The model under review builds one solid part; all positions refer to its coordinate system, in mm. Face numbers are marked on the shaded views. A direction names the side the tool comes from. Round coordinates to 2 decimals unless told otherwise and drop trailing zeros. Order: outer loops, then holes, each group sorted by start corner. A loop starts at its lowest first (then second) coordinate and runs counter-clockwise, first axis right, second up. Notation, with made-up numbers: M -33,-22.5 L 22,-22.5 A24 ccw 22,10.5 Z; hole C 87,19 d5. An arc over 180 degrees is marked long. Answer as a JSON object with one key per item and string values. Group by question number.
1. Add section C-C on y = -5.5. State the section outline as (x, z) points.
2. Add section A-A on x = 8. State the section outline as (y, z) points.
3. Add section D-D on z = -26. State the section outline as (x, y) points, and give its area (3 significant figures).
4. Clearance check with flat-ended pins moving along their axes: P1, Ø3, axis at x = 33, z = -48.5, coming from the -Y side; P2, Ø6.5, axis at x = 76.5, z = -55.5, coming from the -Y side; P3, Ø2, axis at x = 25, y = 2, coming from the +Z side. State where each tip first meets the part, or that it passes through.
5. Add section B-B on y = 3.5. State the section outline as (x, z) points.
6. Machinability: for the marked faces 1 and 2, which of the approach directions +Z, -Z, +X, -X, +Y, -Y give a long, thin tool a straight path to every point of the face, cutting with its end or side? Answer none if there is none.
7. To check wall thickness, follow probe 1 along Z at (x, y) = (42, 4); probe 2 along Y at (x, z) = (53, -52); probe 3 along X at (y, z) = (0.5, -25.5). State the ranges of each line that lie inside material, in increasing order. Write a range as [from, to].
Autodesk Inventor part; units mm, degrees
ref_plane "YZ Plane" through (0, 0, 0) normal (1, 0, 0) x (0, 1, 0)
ref_plane "XZ Plane" through (0, 0, 0) normal (0, 1, 0) x (-1, 0, 0)
ref_plane "XY Plane" through (0, 0, 0) normal (0, 0, 1) x (1, 0, 0)
sketch "Boceto1" plane through (0, 0, 0) normal (0, 1, 0) x (-1, 0, 0)
  line L0 (0, -100) -> (0, 0)
  line L1 (-76, -48) -> (-24, -48)
  line L2 (-24, -64) -> (-76, -64)
  arc A0 (-16, -100) -> (0, -100) centre (-8, -100) ccw
  arc A1 (0, 0) -> (-16, 0) centre (-8, 0) ccw
  arc A2 (-76, -48) -> (-76, -64) centre (-76, -56) ccw
  line L3 (-16, 0) -> (-16, -40)
  line L4 (-16, -72) -> (-16, -100)
  arc A3 (-24, -48) -> (-16, -40) centre (-24, -40) ccw
  arc A4 (-16, -72) -> (-24, -64) centre (-24, -72) ccw
  circle A5 centre (-8, 0) radius 4
  circle A6 centre (-8, -100) radius 4
  circle A7 centre (-76, -56) radius 4
  circle A8 centre (-76, -58) radius 0.5
  circle A9 centre (-76, -54) radius 0.5
  circle A10 centre (-8, -100) radius 2
  circle A11 centre (-8, 0) radius 2
  point P0 (-16, -48)
  dimension "d0" = 16
  dimension "d1" = 100
  dimension "d2" = 60
  dimension "d3" = 16
  dimension "d6" = 8
  dimension "d7" = 8
  dimension "d8" = 8
  dimension "d9" = 8
  dimension "d10" = 8
  dimension "d11" = 8
  dimension "d12" = 8
  dimension "d13" = 1
  dimension "d14" = 1
  dimension "d15" = 2
  dimension "d16" = 2
  dimension "d17" = 4
  dimension "d18" = 4
extrude "Extrusión1" add sketch "Boceto1" along normal blind 5 contours A0 L4 A4 L2 A2 L1 A3 L3 A1 L0 | A5 | A6 | A7 | A8 | A9 | A10 | A11
sketch "Boceto4" plane through (0, 0, 0) normal (0, -1, 0) x (1, 0, 0)
  point P0 (0, 0)
extrude "Extrusión3" add sketch "Boceto1" against normal blind 14 contours A10 | A11
sketch "Boceto5" plane through (0, 0, 0) normal (0, -1, 0) x (1, 0, 0)
  point P0 (0, 0)
extrude "Extrusión4" add sketch "Boceto1" against normal blind 12 contours A8 | A9
sketch "Boceto6" plane through (0, 0, 0) normal (0, -1, 0) x (1, 0, 0)
  point P0 (0, 0)
extrude "Extrusión5" add sketch "Boceto1" against normal blind 10 contours A5 | A6 | A7 | A10 | A11
properties part number "Practica 8"
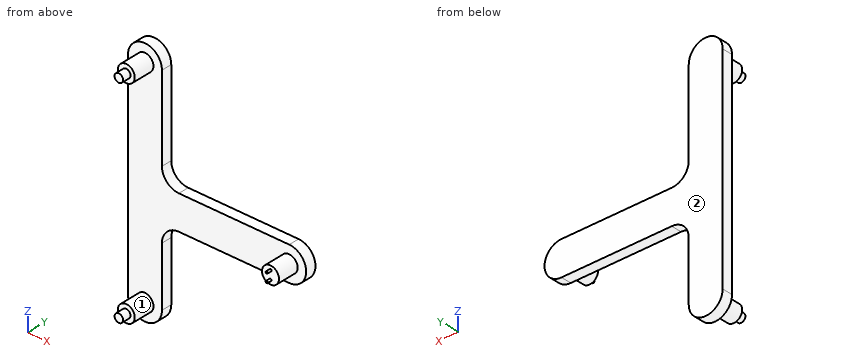
Recorded:
{
 "1": {"outline": "C 8,-100 d8; C 8,0 d8; C 76,-56 d8"},
 "2": {"outline": "M -14,-102 L -10,-102 L -10,-104 L 0,-104 L 0,-108 L 5,-108 L 5,8 L 0,8 L 0,4 L -10,4 L -10,2 L -14,2 L -14,-2 L -10,-2 L -10,-4 L 0,-4 L 0,-96 L -10,-96 L -10,-98 L -14,-98 Z"},
 "3": {"outline": "M 0,0 L 16,0 L 16,5 L 0,5 Z", "area": "80.0 mm²"},
 "4": {"P1": "stops at y = 0", "P2": "stops at y = -12", "P3": "stops at z = -48"},
 "5": {"outline": "M 0,-100 A8 ccw 16,-100 L 16,-72 A8 cw 24,-64 L 76,-64 A8 ccw 76,-48 L 24,-48 A8 cw 16,-40 L 16,0 A8 ccw 0,0 Z"},
 "6": {"face 1": "-Y", "face 2": "+Z, -Z, +X, -X, +Y"},
 "7": {"probe 1": "z = [-64, -48]", "probe 2": "y = [0, 5]", "probe 3": "x = [0, 16]"}
}
